Check sheet for the drawn part. Datum: minimum x, y, z corner. Units: mm. Give positions to 0.01 mm unless a question says otherwise; leave off trailing zeros. Loops run counter-clockwise (first coordinate to the right, second up) from the corner with the lowest first, then second, coordinate; pieces in that order, holes last. Notation, with made-up numbers: (52.5, 63.25) - (96.5, 63.25) arc R15 cw to (96.5, 90.25) - close; hole circle Ø9 at (64.25, -32.75). An arc over 180 degrees is marked (long way). Use a Markdown table: item, result. Add a question column.
1. Material ranges on L1, parallel to Y at x = 97.4, z = 9.2; L2, parallel to X at y = 34.5, z = 7.25; L3, parallel to X at y = 37, z = 5, recorded low to high.
2. Cross-section at A-A on x = 57.5. Enter the section's corners in (y, z), and give its area (3 significant figures).
3. Cross-section at C-C on x = 97.4. Enter the section's corners in (y, z).
4. Cross-section at B-B on y = 67.5. Enter the section's corners in (x, z), and give its area (3 significant figures).
5. Depth check by flat-ended pin: P1, Ø8, axis at x = 17.6, y = 37.5, coming from the -Z side; P2, Ø3, axis at x = 17, y = 68.5, coming from the +Z side. Enter the tip coordinate at first touch or a pass-through.
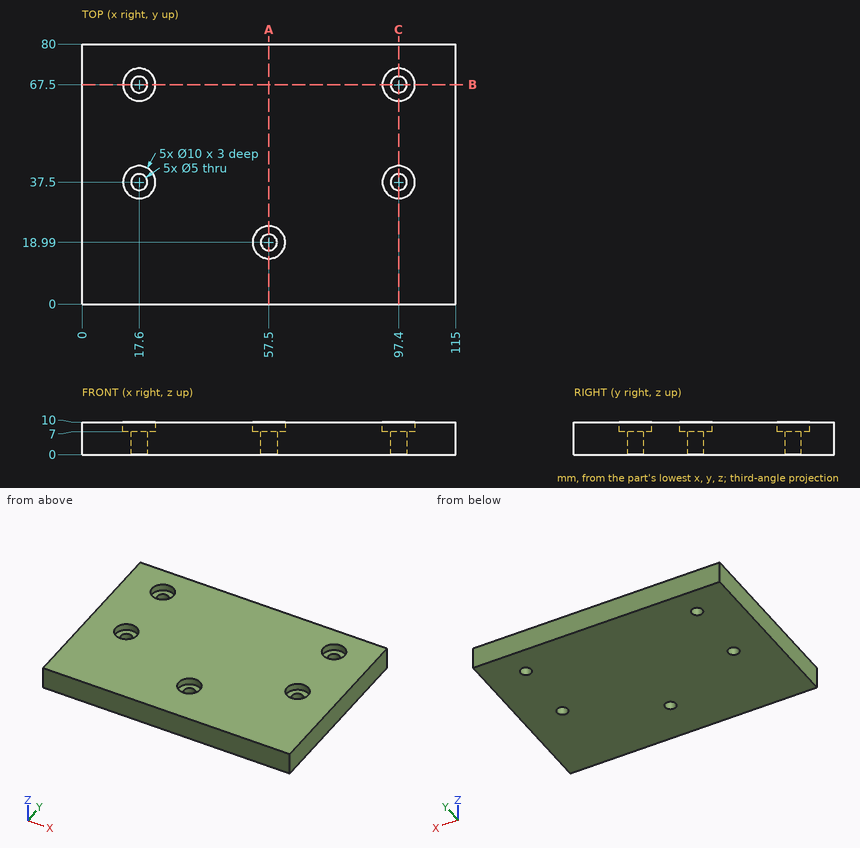
Values found:
| question | item | result |
|---|---|---|
| 1 | L1 | y = 0 to 32.5, 42.5 to 62.5, 72.5 to 80 |
| 1 | L2 | x = 0 to 13.6, 21.6 to 93.4, 101.4 to 115 |
| 1 | L3 | x = 0 to 15.15, 20.05 to 94.95, 99.85 to 115 |
| 2 | outline | (0, 0) - (16.49, 0) - (16.49, 7) - (13.99, 7) - (13.99, 10) - (0, 10) - close; (21.49, 0) - (80, 0) - (80, 10) - (23.99, 10) - (23.99, 7) - (21.49, 7) - close |
| 2 | area | 735 mm2 |
| 3 | outline | (0, 0) - (35, 0) - (35, 7) - (32.5, 7) - (32.5, 10) - (0, 10) - close; (40, 0) - (65, 0) - (65, 7) - (62.5, 7) - (62.5, 10) - (42.5, 10) - (42.5, 7) - (40, 7) - close; (70, 0) - (80, 0) - (80, 10) - (72.5, 10) - (72.5, 7) - (70, 7) - close |
| 4 | outline | (0, 0) - (15.1, 0) - (15.1, 7) - (12.6, 7) - (12.6, 10) - (0, 10) - close; (20.1, 0) - (94.9, 0) - (94.9, 7) - (92.4, 7) - (92.4, 10) - (22.6, 10) - (22.6, 7) - (20.1, 7) - close; (99.9, 0) - (115, 0) - (115, 10) - (102.4, 10) - (102.4, 7) - (99.9, 7) - close |
| 4 | area | 1,020 mm2 |
| 5 | P1 | stops at z = 0 |
| 5 | P2 | stops at z = 7 |
